```python
from build123d import *

# Parameters (mm, degrees)
SKETCH2_R           = 2.5
BOSS_EXTRUDE2_DEPTH = 22.2
FILLET1_R           = 0.5


with BuildPart() as part:
    # Sketch2 → Boss-Extrude2 (new body)
    with BuildSketch(Plane.XY):
        with BuildLine():
            Line((4.955, 19.4), (-4.955, 19.4))
            Line((-4.955, 19.4), (-6.285688199, 24.609959851))
            ThreePointArc((-6.285688199, 24.609959851), (-15.580492928, -20.060115656), (25.4, 0))
            ThreePointArc((25.4, 0), (20.060115656, 15.580492928), (6.285688199, 24.609959851))
            Line((6.285688199, 24.609959851), (4.955, 19.4))
        make_face()
        Circle(SKETCH2_R, mode=Mode.SUBTRACT)
    extrude(amount=BOSS_EXTRUDE2_DEPTH)

    # Fillet1
    fillet1_edges = [part.edges().sort_by_distance(p)[0] for p in [
        (-4.955, 19.4, 11.1),
        (4.955, 19.4, 11.1),
        (6.285688199, 24.609959851, 11.1),
        (-6.285688199, 24.609959851, 11.1),
    ]]
    fillet(fillet1_edges, radius=FILLET1_R)


solid = part.part
```
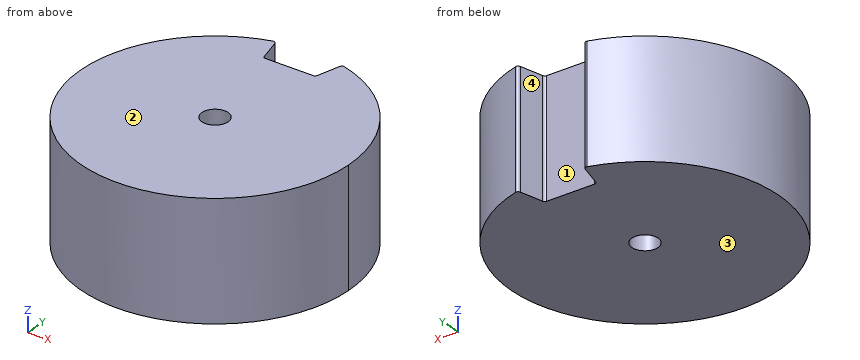
Could you check a few things on this model? Use its own coordinates, in mm. Face numbers are marked on the shaded views. A direction names the side the tool comes from. Round coordinates to 2 decimals unless told otherwise and drop trailing zeros. Order: outer loops, then holes, each group sorted by start corner. A loop starts at its lowest first (then second) coordinate and runs counter-clockwise, first axis right, second up. Notation, with made-up numbers: M 73.25,69 L 104.25,69 A11 ccw 104.25,82 Z; hole C 50,-9.75 d10. An arc over 180 degrees is marked long. One line per question, with ' | ' between items. Start each with the question number.
(1) For the marked faces 3 and 4, which set-ups out of +Z, -Z, +X, -X, +Y, -Y let a thin tool reach every point of the face, with its end or its side?
(2) Please list where these lines run through material, in increasing order: line 1 along Y through (x, z) = (0, 12.75); line 2 along Y through (x, z) = (1.5, 6.25); line 3 along X through (y, z) = (10, 14).
(3) For P1, Ø6, axis at x = -14.5, z = 15, coming from the +Y side; P2, Ø5, axis at x = -9, z = 7, coming from the -Y side; P3, Ø6, axis at y = 5, z = 13, coming from the +X side, each with a flat end and sliding along its axis, tell me the tip position at first contact or that it passes through.
(4) Suppose I cut it at D-D on x = -10.5. List the corners of the cut face in (y, z) for me, then the cut area to 3 significant figures.
(5) Thinking about a two-plate mould opening in X: for the marked faces 1 and 2, which applies, +X half, -X half, draft (parallel to the pull), parting line (faces both ways), or undercut?
(6) Suppose I cut it at C-C on y = -14. List the corners of the cut face in (x, z) for me, then the cut area to 3 significant figures.
(7) Suppose I cut it at B-B on x = 0. List the corners of the cut face in (y, z) for me, then the cut area to 3 significant figures.
(8) Suppose I cut it at A-A on z = 9.5. List the corners of the cut face in (x, y) for me, then the cut area to 3 significant figures.
Geometry results:
1) face 3: -Z, +X, -X, +Y, -Y | face 4: +Z, -Z, +Y
2) line 1: -25.4 to -2.5, 2.5 to 19.4 | line 2: -25.36 to -2, 2 to 19.4 | line 3: -23.35 to 23.35
3) P1: y = 22.65 | P2: y = -24.55 | P3: x = 25.32
4) outline: M -23.13,0 L 23.13,0 L 23.13,22.2 L -23.13,22.2 Z | area: 1,030 mm²
5) face 1: undercut | face 2: draft
6) outline: M -21.19,0 L 21.19,0 L 21.19,22.2 L -21.19,22.2 Z | area: 941 mm²
7) outline: M -25.4,0 L -2.5,0 L -2.5,22.2 L -25.4,22.2 Z; M 2.5,0 L 19.4,0 L 19.4,22.2 L 2.5,22.2 Z | area: 884 mm²
8) outline: M -6.78,24.48 A25.4 ccw long 6.78,24.48 A0.5 ccw 6.16,24.12 L 5.05,19.78 A0.5 cw 4.57,19.4 L -4.57,19.4 A0.5 cw -5.05,19.78 L -6.16,24.12 A0.5 ccw Z; hole C 0,0 d5 | area: 1,940 mm²
